Work out the finished part from the listing and answer in its coordinate system (mm). Give positions to 0.01 mm unless a question says otherwise; leave off trailing zeros. Write each loop counter-clockwise with the first axis right and the second up, starting at its lowest first coordinate (ties: lowest second). Pieces come first, ordered by that corner, then holes. Notation, with made-up numbers: (9.5, 22) - (65.5, 22) arc R12 cw to (65.5, 40) - close; hole circle Ø10 at (-9.75, 63.5). An arc over 180 degrees is marked (long way). Write item = value, one per line.
from build123d import *

# Parameters (mm, degrees)
CYLINDER001_R     = 1.75
CYLINDER001_DEPTH = 3
CYLINDER_R        = 2.75
CYLINDER_DEPTH    = 3


with BuildPart() as interior:
    # Cylinder001 → Cylinder001 (new body)
    with BuildSketch(Plane.XY):
        Circle(CYLINDER001_R)
    extrude(amount=CYLINDER001_DEPTH)


with BuildPart() as spacer:
    # Cylinder → Cylinder (new body)
    with BuildSketch(Plane.XY):
        Circle(CYLINDER_R)
    extrude(amount=CYLINDER_DEPTH)

    # Cut: cut interior
    add(interior.part, mode=Mode.SUBTRACT)


solid = spacer.part
1. Find section D-D, the plane y = -2.2. Give the vertices of the cut face in (x, z), then the cut area to 3 significant figures.
Solution:
outline = (-1.65, 0) - (1.65, 0) - (1.65, 3) - (-1.65, 3) - close
area = 9.90 mm^2
2. Find section C-C, the plane z = 0.25. Give the vertices of the cut face in (x, y), then the cut area to 3 significant figures.
Solution:
outline = circle Ø5.5 at (0, 0); hole circle Ø3.5 at (0, 0)
area = 14.1 mm^2
3. Find section A-A, the plane x = 0. Give the vertices of the cut face in (y, z).
Solution:
outline = (-2.75, 0) - (-1.75, 0) - (-1.75, 3) - (-2.75, 3) - close; (1.75, 0) - (2.75, 0) - (2.75, 3) - (1.75, 3) - close
4. Given pin 1 (1 mm diameter, centred on x = -1, z = 2, fed in from -Y); pin 2 (1.5 mm diameter, centred on y = -1, z = 2.5, fed in from +X), each flat-ended and moving along its own axis, determine where each tip first touches the part or whether it passes through.
Solution:
pin_1 = -2.7
pin_2 = 2.74
5. Straight lines are drawn through the part: line 1 (Y direction, x = 0, z = 1.3); line 2 (X direction, y = -0.6, z = 0.4). For each, find the intervals that lie inside material, in ascending order.
Solution:
line_1 = -2.75 to -1.75, 1.75 to 2.75
line_2 = -2.68 to -1.64, 1.64 to 2.68
6. For a pull along Y with two mould halves and no side action, classify faces 1 (the cylindrical face through (-0.596, -2.685, 1.479)), 2 (the flat face through (2, 0, 0)), 3 (the cylindrical face through (1.617, -0.67, 1.479)) as pulls with the +Y half, pulls with the -Y half, needs draft (parallel to the pull), parting line crosses it, or undercut.
Solution:
face_1 = parting line crosses it
face_2 = needs draft
face_3 = undercut
